Geometry check sheet. Reference: drawing and pictorial views, mm from the part's lowest x, y, z. A direction names the side the tool comes from. Give positions to 0.01 mm unless a question says otherwise; leave off trailing zeros. Order: outer loops, then holes, each group sorted by start corner. A loop starts at its lowest first (then second) coordinate and runs counter-clockwise, first axis right, second up. Notation, with made-up numbers: M -30.75,-20 L 7.25,-20 A18 ccw 7.25,-14 Z; hole C 35,13 d11. An arc over 180 degrees is marked long. Use CSV: the item, a comma, the result in double quotes. Start each with the question number.
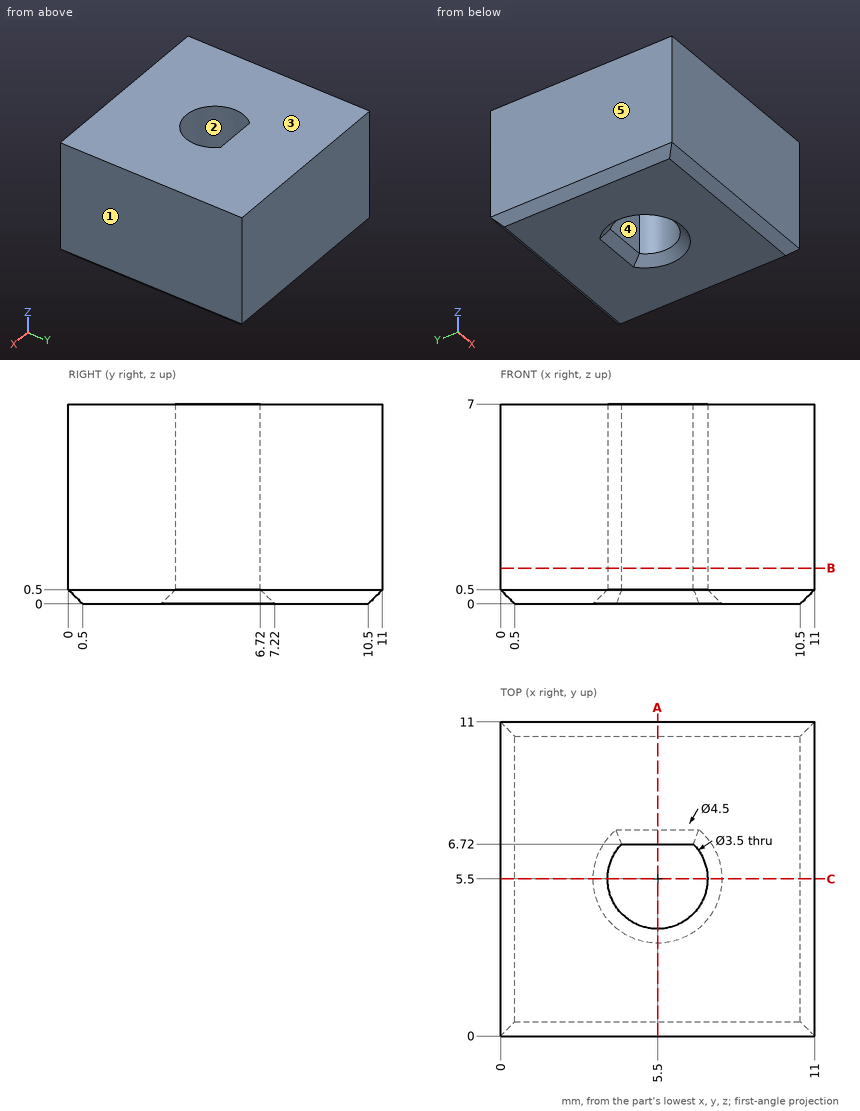
(1) Access from +Z, -Z, +X, -X, +Y, -Y to the whole of each face (thin tool, end or side, straight path). Record for the marked faces 4 and 5.
(2) Thickness scan on line 1 (X direction, y = 5.5, z = 4.5); line 2 (Y direction, x = 5.5, z = 3.25); line 3 (X direction, y = 4.5, z = 3.5). Record the ranges inside material, lowest first.
(3) Sectioned sample at A-A on x = 5.5. Record the cut outline in (y, z), then the cut area to 3 significant figures.
(4) Sectioned sample at B-B on z = 1.25. Record the cut outline in (x, y), then the cut area to 3 significant figures.
(5) Draft check along X on the marked faces 1, 2 and 3. Enter one of: +X half, -X half, draft (parallel to the pull), parting line (faces both ways), or undercut.
(6) Sectioned sample at C-C on y = 5.5. Record the cut outline in (x, z).
Responses:
1,face 4,"+Z, -Z"
1,face 5,"+Z, -Z, -X, +Y, -Y"
2,line 1,"0 to 3.75, 7.25 to 11"
2,line 2,"0 to 3.75, 6.72 to 11"
2,line 3,"0 to 4.06, 6.94 to 11"
3,outline,"M 0,0.5 L 0.5,0 L 3.25,0 L 3.75,0.5 L 3.75,7 L 0,7 Z; M 6.72,0.5 L 7.22,0 L 10.5,0 L 11,0.5 L 11,7 L 6.72,7 Z"
3,area,"55.7 mm2"
4,outline,"M 0,0 L 11,0 L 11,11 L 0,11 Z; hole M 4.25,6.72 A1.75 ccw long 6.75,6.72 Z"
4,area,"112 mm2"
5,face 1,"+X half"
5,face 2,"undercut"
5,face 3,"draft"
6,outline,"M 0,0.5 L 0.5,0 L 3.25,0 L 3.75,0.5 L 3.75,7 L 0,7 Z; M 7.25,0.5 L 7.75,0 L 10.5,0 L 11,0.5 L 11,7 L 7.25,7 Z"
